Here's the drawing with two shaded views (mm, measured from the low corner). I have some questions. A direction names the side the tool comes from. Coordinates: 2 decimals unless noted, no trailing zeros. Loops run counter-clockwise (first coordinate to the right, second up) from the corner with the lowest first, then second, coordinate; pieces in that order, holes last. Notation, with made-up numbers: (18, 24) -> (30, 24) arc R29 cw to (30, 59) -> close; hole circle Ø4 at (87.25, -20.75). An arc over 180 degrees is marked (long way). Answer as a JSON object with one key per item and string values. Group by question number.
Q1. I need wall thicknesses on line 1 (Y direction, x = 28.1, z = 15); line 2 (Z direction, x = 14.75, y = 13.5); line 3 (X direction, y = 21.75, z = 21). Which ranges of each line are inside material? Lowest first, please.
Q2. I want a section at C-C on x = 15. Write out the boundary of the cut face in (y, z) (3 decimals).
Q3. I want a section at A-A on z = 15. Write out the boundary of the cut face in (x, y) (3 decimals), then the cut area to 3 significant figures.
Q4. Thinking about a two-plate mould opening in Z: for the marked faces 1, 2, 3 and 4, which applies, released by +Z, released by -Z, zero draft, split by the parting line, or undercut?
Q5. I want a section at D-D on y = 8.5. Write out the boundary of the cut face in (x, z), then the cut area to 3 significant figures.
Q6. I'm going to push flat-ended pins straight in: pin 1 (5 mm diameter, centred on x = 15, z = 15, fed in from -Y); pin 2 (12 mm diameter, centred on y = 3.5, z = 12, fed in from -X); pin 3 (9 mm diameter, centred on y = 15, z = 15, fed in from +X). Where does each tip first touch, or does it pass through?
Q7. I want a section at B-B on y = 13. Write out the boundary of the cut face in (x, z), then the cut area to 3 significant figures.
Q8. On a 3-axis mill with a long thin cutter (end or side, diameter ignored), from which of +Z, -Z, +X, -X, +Y, -Y can I reach the whole of each face in a straight line? I mean the marked faces 5 and 6. Say none if no direction works.
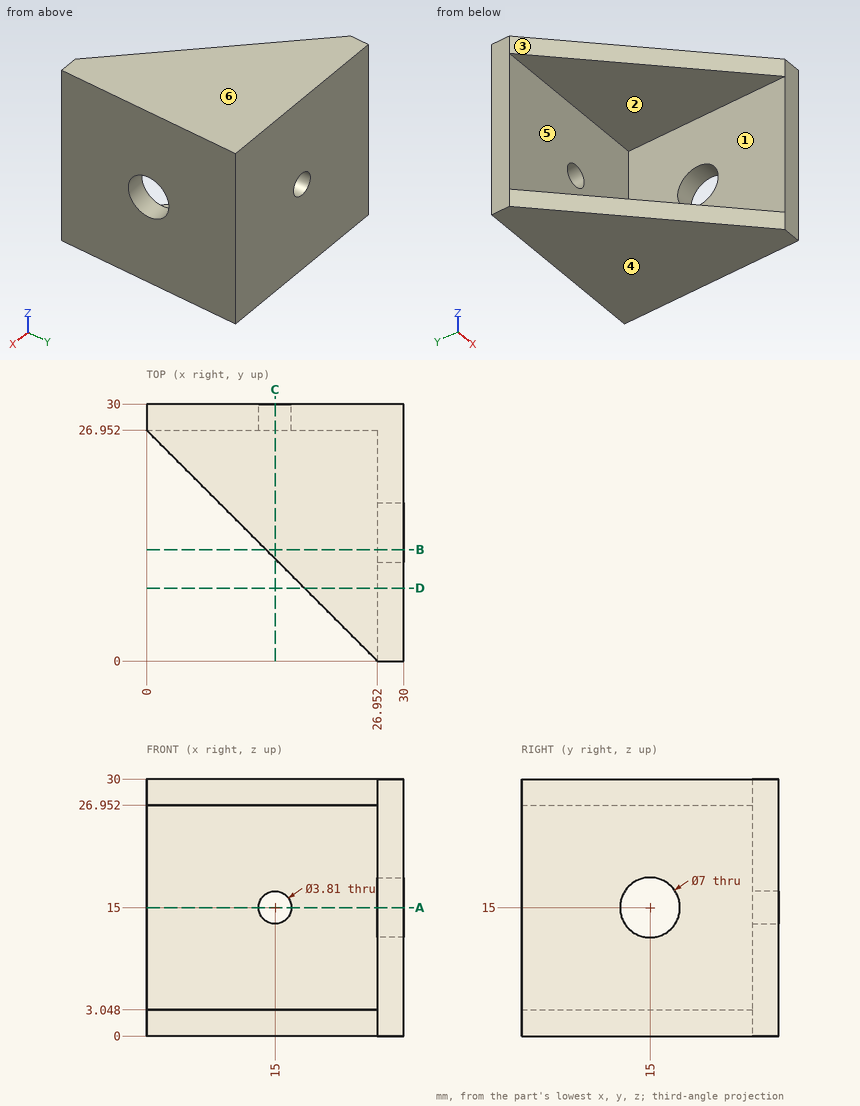
Result set:
{
 "1": {"line 1": "y = 0 to 11.5, 18.5 to 30", "line 2": "z = 0 to 3.05, 26.95 to 30", "line 3": "x = 26.95 to 30"},
 "2": {"outline": "(11.952, 0) -> (30, 0) -> (30, 13.095) -> (26.952, 13.095) -> (26.952, 3.048) -> (11.952, 3.048) -> close; (11.952, 26.952) -> (26.952, 26.952) -> (26.952, 16.905) -> (30, 16.905) -> (30, 30) -> (11.952, 30) -> close"},
 "3": {"outline": "(0, 26.952) -> (13.095, 26.952) -> (13.095, 30) -> (0, 30) -> close; (16.905, 26.952) -> (26.952, 26.952) -> (26.952, 18.5) -> (30, 18.5) -> (30, 30) -> (16.905, 30) -> close; (26.952, 0) -> (30, 0) -> (30, 11.5) -> (26.952, 11.5) -> close", "area": "141 mm²"},
 "4": {"face 1": "undercut", "face 2": "undercut", "face 3": "zero draft", "face 4": "released by -Z"},
 "5": {"outline": "(18.45, 0) -> (30, 0) -> (30, 30) -> (18.45, 30) -> (18.45, 26.95) -> (26.95, 26.95) -> (26.95, 3.05) -> (18.45, 3.05) -> close", "area": "143 mm²"},
 "6": {"pin 1": "stops at y = 26.95", "pin 2": "stops at x = 26.95", "pin 3": "stops at x = 30"},
 "7": {"outline": "(13.95, 0) -> (30, 0) -> (30, 12.13) -> (26.95, 12.13) -> (26.95, 3.05) -> (13.95, 3.05) -> close; (13.95, 26.95) -> (26.95, 26.95) -> (26.95, 17.87) -> (30, 17.87) -> (30, 30) -> (13.95, 30) -> close", "area": "153 mm²"},
 "8": {"face 5": "-X, -Y", "face 6": "+Z, +X, -X, +Y, -Y"}
}
